```python
from build123d import *

# Parameters (mm, degrees)
EXTRUDE_1276_DEPTH          = 10
CUT_EXTRUDE_1340_DEPTH      = 8
EXTRUDE_1406_DEPTH          = 2
CUT_EXTRUDE_1479_DEPTH      = 2
CUT_EXTRUDE_1479_DEPTH_BACK = 2
CUT_EXTRUDE_1550_DEPTH      = 44.279614139
CUT_EXTRUDE_1550_DEPTH_BACK = 44.279614139
SKETCH_1_7_R                = 1
USB_REACH                   = 80.4
USB_2_W                     = 10
USB_2_H                     = 2
CUT_EXTRUDE_START           = -5
SKETCH_3_R                  = 1
CUT_EXTRUDE_3145_DEPTH      = 5
FILLET_3202_R               = 5
CUT_EXTRUDE_3663_DEPTH      = 44.279614288
CUT_EXTRUDE_3663_DEPTH_BACK = 44.279614288
SKETCH_8_W                  = 25.017119527
SKETCH_8_H                  = 8.52
SKETCH_11_W                 = 40
SKETCH_11_H                 = 14
CUT_EXTRUDE_3720_DEPTH      = 9
FILLET_3777_R               = 0.5
CUT_EXTRUDE_12_REACH        = 82.59
USB_4_R                     = 1
CUT_EXTRUDE_4523_DEPTH      = 44.279614288
CUT_EXTRUDE_4523_DEPTH_BACK = 44.279614288
SKETCH_13_R                 = 2.3


with BuildPart() as part:
    # Sketch 378 → Extrude 1276 (new body)
    with BuildSketch(Plane(origin=(0, 0, 0), x_dir=(1, 0, 0), z_dir=(0, 1, 0))):
        with BuildLine():
            Line((-39.25, 12.75), (-39.25, -12.75))
            ThreePointArc((-39.25, -12.75), (-38.517766953, -14.517766953), (-36.75, -15.25))
            Line((-36.75, -15.25), (36.75, -15.25))
            ThreePointArc((36.75, -15.25), (38.517766953, -14.517766953), (39.25, -12.75))
            Line((39.25, -12.75), (39.25, 12.75))
            ThreePointArc((39.25, 12.75), (38.517766953, 14.517766953), (36.75, 15.25))
            Line((36.75, 15.25), (-36.75, 15.25))
            ThreePointArc((-36.75, 15.25), (-38.517766953, 14.517766953), (-39.25, 12.75))
        make_face()
    extrude(amount=EXTRUDE_1276_DEPTH)

    # Эскиз1<3> → Cut-Extrude 1340 (cut)
    with BuildSketch(Plane(origin=(0, 0, 0), x_dir=(1, 0, 0), z_dir=(0, 1, 0))):
        with BuildLine():
            Line((33.968871126, 12), (-33.968871126, 12))
            ThreePointArc((-33.968871126, 12), (-34.818019485, 10.818019485), (-36, 9.968871126))
            Line((-36, 9.968871126), (-36, -9.968871126))
            ThreePointArc((-36, -9.968871126), (-34.818019485, -10.818019485), (-33.968871126, -12))
            Line((-33.968871126, -12), (33.968871126, -12))
            ThreePointArc((33.968871126, -12), (34.818019485, -10.818019485), (36, -9.968871126))
            Line((36, -9.968871126), (36, 9.968871126))
            ThreePointArc((36, 9.968871126), (34.818019485, 10.818019485), (33.968871126, 12))
        make_face()
    extrude(amount=CUT_EXTRUDE_1340_DEPTH, mode=Mode.SUBTRACT)

    # Эскиз1<4> → Extrude 1406 (add)
    with BuildSketch(Plane(origin=(0, 0, 0), x_dir=(1, 0, 0), z_dir=(0, 1, 0))):
        with BuildLine():
            Line((34.645898034, 13), (-34.645898034, 13))
            ThreePointArc((-34.645898034, 13), (-35.525126266, 11.525126266), (-37, 10.645898034))
            Line((-37, 10.645898034), (-37, -10.645898034))
            ThreePointArc((-37, -10.645898034), (-35.525126266, -11.525126266), (-34.645898034, -13))
            Line((-34.645898034, -13), (34.645898034, -13))
            ThreePointArc((34.645898034, -13), (35.525126266, -11.525126266), (37, -10.645898034))
            Line((37, -10.645898034), (37, 10.645898034))
            ThreePointArc((37, 10.645898034), (35.525126266, 11.525126266), (34.645898034, 13))
        make_face()
    extrude(amount=-EXTRUDE_1406_DEPTH)

    # Эскиз1<6> → Cut-Extrude 1479 (cut, two sides: drawn at the far end of the back side and taken through both)
    with BuildSketch(Plane(origin=(0, 0, 0), x_dir=(1, 0, 0), z_dir=(0, 1, 0)).offset(-CUT_EXTRUDE_1479_DEPTH_BACK)):
        with BuildLine():
            Line((33.968871126, 12), (-33.968871126, 12))
            ThreePointArc((-33.968871126, 12), (-34.818019485, 10.818019485), (-36, 9.968871126))
            Line((-36, 9.968871126), (-36, -9.968871126))
            ThreePointArc((-36, -9.968871126), (-34.818019485, -10.818019485), (-33.968871126, -12))
            Line((-33.968871126, -12), (33.968871126, -12))
            ThreePointArc((33.968871126, -12), (34.818019485, -10.818019485), (36, -9.968871126))
            Line((36, -9.968871126), (36, 9.968871126))
            ThreePointArc((36, 9.968871126), (34.818019485, 10.818019485), (33.968871126, 12))
        make_face()
    extrude(amount=CUT_EXTRUDE_1479_DEPTH + CUT_EXTRUDE_1479_DEPTH_BACK, mode=Mode.SUBTRACT)

    # Эскиз1<7> → Cut-Extrude 1550 (cut, two sides: drawn at the far end of the back side and taken through both)
    with BuildSketch(Plane(origin=(0, 0, 0), x_dir=(1, 0, 0), z_dir=(0, 1, 0)).offset(-CUT_EXTRUDE_1550_DEPTH_BACK)):
        with Locations(Location((37.454174909, -13.4, 0), (0, 0, 270))):
            Circle(SKETCH_1_7_R)
        with Locations(Location((-37.4, 13.4, 0), (0, 0, 270))):
            Circle(SKETCH_1_7_R)
        with Locations(Location((37.4, 13.4, 0), (0, 0, 270))):
            Circle(SKETCH_1_7_R)
        with Locations(Location((-37.4, -13.4, 0), (0, 0, 270))):
            Circle(SKETCH_1_7_R)
    extrude(amount=CUT_EXTRUDE_1550_DEPTH + CUT_EXTRUDE_1550_DEPTH_BACK, mode=Mode.SUBTRACT)

    # USB 2 → USB (cut, up to next)
    with BuildSketch(Plane.ZY.offset(37), mode=Mode.PRIVATE) as usb_sk1:
        with Locations((0, -1)):
            Rectangle(USB_2_W, USB_2_H)
    usb_tool1 = extrude(usb_sk1.sketch, amount=-USB_REACH, mode=Mode.PRIVATE) & part.part
    add(usb_tool1.solids().sort_by_distance((-37, -1, 0))[0], mode=Mode.SUBTRACT)

    # Эскиз3 → Cut-Extrude 3145 (cut)
    # profile 1 of 4: a face of its own
    with BuildSketch(Plane(origin=(0, 10, 0), x_dir=(1, 0, 0), z_dir=(0, 1, 0)).offset(CUT_EXTRUDE_START)):
        with BuildLine():
            Line((-34.4, 13.4), (-34.4, 15.25))
            Line((-34.4, 15.25), (-36.75, 15.25))
            ThreePointArc((-36.75, 15.25), (-38.517766953, 14.517766953), (-39.25, 12.75))
            Line((-39.25, 12.75), (-39.25, 10.4))
            Line((-39.25, 10.4), (-37.4, 10.4))
            ThreePointArc((-37.4, 10.4), (-35.278679656, 11.278679656), (-34.4, 13.4))
        make_face()
        with Locations(Location((-37.4, 13.4, 0), (0, 0, 270))):
            Circle(SKETCH_3_R, mode=Mode.SUBTRACT)
    # profile 2 of 4: a face of its own
    with BuildSketch(Plane(origin=(0, 10, 0), x_dir=(1, 0, 0), z_dir=(0, 1, 0)).offset(CUT_EXTRUDE_START)):
        with BuildLine():
            Line((-36.75, -15.25), (-34.4, -15.25))
            Line((-34.4, -15.25), (-34.4, -13.4))
            ThreePointArc((-34.4, -13.4), (-35.278679656, -11.278679656), (-37.4, -10.4))
            Line((-37.4, -10.4), (-39.25, -10.4))
            Line((-39.25, -10.4), (-39.25, -12.75))
            ThreePointArc((-39.25, -12.75), (-38.517766953, -14.517766953), (-36.75, -15.25))
        make_face()
        with Locations(Location((-37.4, -13.4, 0), (0, 0, 270))):
            Circle(SKETCH_3_R, mode=Mode.SUBTRACT)
    # profile 3 of 4: a face of its own
    with BuildSketch(Plane(origin=(0, 10, 0), x_dir=(1, 0, 0), z_dir=(0, 1, 0)).offset(CUT_EXTRUDE_START)):
        with BuildLine():
            ThreePointArc((36.75, -15.25), (38.517766953, -14.517766953), (39.25, -12.75))
            Line((39.25, -12.75), (39.25, -10.4))
            Line((39.25, -10.4), (37.454174909, -10.4))
            ThreePointArc((37.454174909, -10.4), (35.332854565, -11.278679656), (34.454174909, -13.4))
            Line((34.454174909, -13.4), (34.454174909, -15.25))
            Line((34.454174909, -15.25), (36.75, -15.25))
        make_face()
        with Locations(Location((37.454174909, -13.4, 0), (0, 0, 270))):
            Circle(SKETCH_3_R, mode=Mode.SUBTRACT)
    # profile 4 of 4: a face of its own
    with BuildSketch(Plane(origin=(0, 10, 0), x_dir=(1, 0, 0), z_dir=(0, 1, 0)).offset(CUT_EXTRUDE_START)):
        with BuildLine():
            Line((37.4, 10.4), (39.25, 10.4))
            Line((39.25, 10.4), (39.25, 12.75))
            ThreePointArc((39.25, 12.75), (38.517766953, 14.517766953), (36.75, 15.25))
            Line((36.75, 15.25), (34.4, 15.25))
            Line((34.4, 15.25), (34.4, 13.4))
            ThreePointArc((34.4, 13.4), (35.278679656, 11.278679656), (37.4, 10.4))
        make_face()
        with Locations(Location((37.4, 13.4, 0), (0, 0, 270))):
            Circle(SKETCH_3_R, mode=Mode.SUBTRACT)
    extrude(amount=CUT_EXTRUDE_3145_DEPTH, mode=Mode.SUBTRACT)

    # Fillet 3202
    # the kernel refuses this fillet: 5 mm, written as the material it takes off along each edge
    with BuildSketch(Plane(origin=(-39.25, 10, -22.9), x_dir=(0, -1, 0), z_dir=(0, 0, 1)), Plane(origin=(39.25, 10, 22.9), x_dir=(0, -1, 0), z_dir=(0, 0, -1))) as fillet_3202_piece_1:
        with BuildLine():
            CenterArc((FILLET_3202_R, FILLET_3202_R), FILLET_3202_R, 180, 90)
            Line((0, FILLET_3202_R), (0, 0))
            Line((0, 0), (FILLET_3202_R, 0))
        make_face()
    extrude(amount=45.8, mode=Mode.SUBTRACT)
    with BuildSketch(Plane(origin=(46.9, 10, -15.25), x_dir=(0, -1, 0), z_dir=(-1, 0, 0))) as fillet_3202_piece_2:
        with BuildLine():
            CenterArc((FILLET_3202_R, FILLET_3202_R), FILLET_3202_R, 180, 90)
            Line((0, FILLET_3202_R), (0, 0))
            Line((0, 0), (FILLET_3202_R, 0))
        make_face()
    extrude(amount=93.8, mode=Mode.SUBTRACT)
    with BuildSketch(Plane(origin=(-46.9, 10, 15.25), x_dir=(0, -1, 0), z_dir=(1, 0, 0))) as fillet_3202_piece_3:
        with BuildLine():
            CenterArc((FILLET_3202_R, FILLET_3202_R), FILLET_3202_R, 180, 90)
            Line((0, FILLET_3202_R), (0, 0))
            Line((0, 0), (FILLET_3202_R, 0))
        make_face()
    extrude(amount=93.854174909, mode=Mode.SUBTRACT)

    # основной эскиз<8> → Cut-Extrude 3663 (cut, two sides: drawn at the far end of the back side and taken through both)
    with BuildSketch(Plane(origin=(0, 0, 0), x_dir=(1, 0, 0), z_dir=(0, 1, 0)).offset(-CUT_EXTRUDE_3663_DEPTH_BACK)):
        with Locations((-1.813623337, 1.023507904)):
            Rectangle(SKETCH_8_W, SKETCH_8_H)
    extrude(amount=CUT_EXTRUDE_3663_DEPTH + CUT_EXTRUDE_3663_DEPTH_BACK, mode=Mode.SUBTRACT)

    # основной эскиз<11> → Cut-Extrude 3720 (cut)
    with BuildSketch(Plane(origin=(0, 0, 0), x_dir=(1, 0, 0), z_dir=(0, 1, 0))):
        with Locations((-0.9221831, -0.056492096)):
            Rectangle(SKETCH_11_W, SKETCH_11_H)
    extrude(amount=CUT_EXTRUDE_3720_DEPTH, mode=Mode.SUBTRACT)

    # Fillet 3777
    fillet_3777_edges = [part.edges().sort_by_distance(p)[0] for p in [
        (10.694936427, 10, -1.023507904),
        (-1.813623336, 10, -5.283507904),
        (-14.3221831, 10, -1.023507904),
        (-1.813623336, 10, 3.236492096),
    ]]
    fillet(fillet_3777_edges, radius=FILLET_3777_R)

    # USB 3 → Вырез-Вытянуть12 (cut, up to next)
    with BuildSketch(Plane.ZY.offset(39.25), mode=Mode.PRIVATE) as cut_extrude_12_sk1:
        Polygon((-4.125, -0.7), (4.125, -0.7), (4.125, 0), (3.635102051, 0.8), (-3.635102051, 0.8), (-4.125, 0), align=None)
    cut_extrude_12_tool1 = extrude(cut_extrude_12_sk1.sketch, amount=-CUT_EXTRUDE_12_REACH, mode=Mode.PRIVATE) & part.part
    add(cut_extrude_12_tool1.solids().sort_by_distance((-39.25, 0.034192, 0))[0], mode=Mode.SUBTRACT)

    # USB 4
    usb_4_edges = [part.edges().sort_by_distance(p)[0] for p in [
        (-37.625, 0.8, 3.635102051),
        (-37.625, 0.8, -3.635102051),
    ]]
    fillet(usb_4_edges, radius=USB_4_R)

    # основной эскиз<13> → Cut-Extrude 4523 (cut, two sides: drawn at the far end of the back side and taken through both)
    with BuildSketch(Plane(origin=(0, 0, 0), x_dir=(1, 0, 0), z_dir=(0, 1, 0)).offset(-CUT_EXTRUDE_4523_DEPTH_BACK)):
        with Locations(Location((27.584507944, 8.749878541, 0), (0, 0, 270))):
            Circle(SKETCH_13_R)
        with Locations(Location((30.584507944, -0.000121459, 0), (0, 0, 270))):
            Circle(SKETCH_13_R)
        with Locations(Location((27.584507944, -8.750117644, 0), (0, 0, 270))):
            Circle(SKETCH_13_R)
    extrude(amount=CUT_EXTRUDE_4523_DEPTH + CUT_EXTRUDE_4523_DEPTH_BACK, mode=Mode.SUBTRACT)


solid = part.part
```
CAD build for the part. Positions are in the model's coordinates, mm. A direction names the side the tool comes from. Coordinates: 2 decimals unless noted, no trailing zeros. Write each loop counter-clockwise with the first axis right and the second up, starting at its lowest first coordinate (ties: lowest second). Pieces come first, ordered by that corner, then holes.
(1) Two-plate mould, pull along Z, no slides. Class faces 5 (the face through (-35.26, 7.41, 11.3)), 6 (the face through (34.833, 2.93, -10.804)), 7 (the face through (38, 6, -10.4)): +Z half, -Z half, draft (parallel to the pull), parting line (faces both ways), or undercut.
(2) Flat gauge pins, fed straight in: pin 1 (12 mm diameter, centred on x = -4, z = 0, fed in from -Y); pin 2 (3 mm diameter, centred on x = 26, z = -7.5, fed in from +Y); pin 3 (0.6 mm diameter, centred on y = 7, z = -14.5, fed in from +X); pin 4 (1 mm diameter, centred on y = -1.5, z = -4, fed in from +X). Where does each tip first touch, or does it go through?
(3) Drill centre lines: probe 1 along Z at (x, y) = (14.5, -0.5); probe 2 along X at (y, z) = (1.8, 13.4); probe 3 along X at (y, z) = (1.25, 13). Where is each one in solid material? Low to high.
(4) 3-axis set-ups, long thin cutter, end or side, ignore diameter. For faces 1 (the face through (34.4, 6, -14)), 2 (the face through (-34.804, 2.93, -10.833)), 3 (the face through (37, -1, 0)), 4 (the face through (38, 6, 10.4)): which of +Z, -Z, +X, -X, +Y, -Y reach the whole face in a straight line?
(5) Cut at D-D, the plane x = -26. List the corners of the cut face in (y, z), and give its area (3 significant figures).
(6) Cut at A-A, the plane x = -7.5. List the corners of the cut face in (y, z).
(7) Cut at B-B, the plane y = 1.5. List the corners of the cut face in (x, z), and give its area (3 significant figures).
(8) Cut at C-C, the plane z = 9. List the corners of the cut face in (x, y), and give its area (3 significant figures).
Geometry says:
1. face 5: +Z half
1. face 6: undercut
1. face 7: -Z half
2. pin 1: stops at y = 9
2. pin 2: stops at y = 10
2. pin 3: stops at x = 34.4
2. pin 4: stops at x = 37
3. probe 1: z = -13 to -12, 12 to 13
3. probe 2: x = -39.16 to -38.4, -36.4 to 36.45, 38.45 to 39.16
3. probe 3: x = -39.24 to -38.32, -36.48 to 36.54, 38.37 to 39.24
4. face 1: -Z, +X, +Y
4. face 2: -Y
4. face 3: +Z, -Z, +X, -Y
4. face 4: +Z, +X, +Y
5. outline: (-2, -13) - (0, -13) - (0, -15.25) - (5, -15.25) arc R5 ccw to (10, -10.25) - (10, 10.25) arc R5 ccw to (5, 15.25) - (0, 15.25) - (0, 13) - (-2, 13) - (-2, 12) - (8, 12) - (8, -12) - (-2, -12) - close
5. area: 106 mm2
6. outline: (-2, -13) - (0, -13) - (0, -15.25) - (5, -15.25) arc R5 ccw to (10, -10.25) - (10, -5.78) arc R0.5 ccw to (9.5, -5.28) - (9, -5.28) - (9, -6.94) - (8, -6.94) - (8, -12) - (-2, -12) - close; (-2, 12) - (8, 12) - (8, 7.06) - (9, 7.06) - (9, 3.24) - (9.5, 3.24) arc R0.5 ccw to (10, 3.74) - (10, 10.25) arc R5 ccw to (5, 15.25) - (0, 15.25) - (0, 13) - (-2, 13) - close
7. outline: (-39.25, -12.75) arc R2.5 ccw to (-36.75, -15.25) - (36.75, -15.25) arc R2.5 ccw to (39.25, -12.75) - (39.25, 12.75) arc R2.5 ccw to (36.75, 15.25) - (-36.75, 15.25) arc R2.5 ccw to (-39.25, 12.75) - close; hole circle Ø2 at (-37.4, -13.4); hole circle Ø2 at (-37.4, 13.4); hole (-36, -9.97) arc R4.5 cw to (-33.97, -12) - (33.97, -12) arc R4.5 cw to (36, -9.97) - (36, 9.97) arc R4.5 cw to (33.97, 12) - (-33.97, 12) arc R4.5 cw to (-36, 9.97) - close; hole circle Ø2 at (37.4, -13.4); hole circle Ø2 at (37.45, 13.4)
7. area: 658 mm2
8. outline: (-39.25, 0) - (-37, 0) - (-37, -2) - (-36, -2) - (-36, 8) - (25.3, 8) - (25.3, 10) - (-34.25, 10) arc R5 ccw to (-39.25, 5) - close; (29.87, 8) - (36, 8) - (36, -2) - (37, -2) - (37, 0) - (39.25, 0) - (39.25, 5) arc R5 ccw to (34.25, 10) - (29.87, 10) - close
8. area: 193 mm2
